CAD build for the part. Positions are in the model's coordinates, mm. A direction names the side the tool comes from. Round coordinates to 2 decimals unless told otherwise and drop trailing zeros. Loops run counter-clockwise (first coordinate to the right, second up) from the corner with the lowest first, then second, coordinate; pieces in that order, holes last. Notation, with made-up numbers: (-3, 39) - (30, 39) arc R20 cw to (30, 55) - close; hole circle Ø11 at (1, 65.5). An arc over 180 degrees is marked (long way). One line per question, with ' | ' between items.
```python
from build123d import *

# Parameters (mm, degrees)
SKETCH1_W                                      = 200
SKETCH1_H                                      = 174.75
BOSS_EXTRUDE1_DEPTH                            = 25
SKETCH2_W                                      = 40
SKETCH2_H                                      = 9.75
CUT_EXTRUDE1_DEPTH                             = 19.8
SKETCH3_W                                      = 37.5
SKETCH3_H                                      = 60
CUT_EXTRUDE2_DEPTH                             = 26
BOSS_EXTRUDE2_DEPTH                            = 25
SKETCH5_R                                      = 1.65
CUT_EXTRUDE3_DEPTH                             = 1.23
SKETCH6_R                                      = 3.325
CUT_EXTRUDE4_DEPTH                             = 26
SKETCH7_R                                      = 0.685
CUT_EXTRUDE5_DEPTH                             = 6.2
F_1_4_20_TAPPED_HOLE1_D                        = 5.1054
CBORE_FOR_4_SOCKET_HEAD_CAP_SCREW1_D           = 3.2639
CBORE_FOR_4_SOCKET_HEAD_CAP_SCREW1_CBORE_D     = 5.55752
CBORE_FOR_4_SOCKET_HEAD_CAP_SCREW1_CBORE_DEPTH = 2.8448


with BuildPart() as part:
    # Sketch1 → Boss-Extrude1 (new body)
    with BuildSketch(Plane(origin=(0, 0, 0), x_dir=(1, 0, 0), z_dir=(0, 1, 0))):
        Rectangle(SKETCH1_W, SKETCH1_H)
    extrude(amount=BOSS_EXTRUDE1_DEPTH)

    # Sketch2 → Cut-Extrude1 (cut)
    with BuildSketch(Plane(origin=(0, 25, 0), x_dir=(1, 0, 0), z_dir=(0, 1, 0))):
        with Locations((-80, -82.5)):
            Rectangle(SKETCH2_W, SKETCH2_H)
    extrude(amount=-CUT_EXTRUDE1_DEPTH, mode=Mode.SUBTRACT)

    # Sketch3 → Cut-Extrude2 (cut, through all)
    with BuildSketch(Plane(origin=(0, 25, 0), x_dir=(1, 0, 0), z_dir=(0, 1, 0))):
        with Locations((-79.98, -42.625)):
            Rectangle(SKETCH3_W, SKETCH3_H)
        Polygon((-25, -42.625), (100, -42.625), (100, -87.375), (-60, -87.375), (-60, -12.625), (-25, -12.625), align=None)
    extrude(amount=-CUT_EXTRUDE2_DEPTH, mode=Mode.SUBTRACT)

    # Sketch4 → Boss-Extrude2 (add)
    with BuildSketch(Plane(origin=(0, 25, 0), x_dir=(1, 0, 0), z_dir=(0, 1, 0))):
        Polygon((-60, -74.625), (-5.5, -74.625), (-5.5, -73.455), (-50.1, -73.455), (-50.1, -69.865), (49.9, -69.865), (49.9, -73.455), (5.2, -73.455), (5.2, -74.625), (59.7, -74.625), (59.7, -75.855), (5.2, -75.855), (5.2, -77.025), (49.9, -77.025), (49.9, -80.615), (-50.1, -80.615), (-50.1, -77.025), (-5.5, -77.025), (-5.5, -75.855), (-60, -75.855), align=None)
        Polygon((-3.1, -72.225), (-3.1, -78.255), (-47.63, -78.255), (-47.63, -79.385), (47.43, -79.385), (47.43, -78.255), (2.8, -78.255), (2.8, -72.225), (47.43, -72.225), (47.43, -71.095), (-47.63, -71.095), (-47.63, -72.225), align=None, mode=Mode.SUBTRACT)
    extrude(amount=-BOSS_EXTRUDE2_DEPTH)

    # Sketch5 → Cut-Extrude3 (cut)
    with BuildSketch(Plane.XY.offset(75.855)):
        with Locations((54.55, 12.65)):
            Circle(SKETCH5_R)
    extrude(amount=-CUT_EXTRUDE3_DEPTH, mode=Mode.SUBTRACT)

    # Sketch6 → Cut-Extrude4 (cut, through all)
    with BuildSketch(Plane(origin=(0, 25, 0), x_dir=(1, 0, 0), z_dir=(0, 1, 0))):
        with Locations((-80.175, 67.55)):
            Circle(SKETCH6_R)
        with Locations((-4.025, 67.55)):
            Circle(SKETCH6_R)
        with Locations((-4.025, 16.9)):
            Circle(SKETCH6_R)
    extrude(amount=-CUT_EXTRUDE4_DEPTH, mode=Mode.SUBTRACT)

    # Sketch7 → Cut-Extrude5 (cut, through all)
    with BuildSketch(Plane(origin=(0, 5.2, 0), x_dir=(1, 0, 0), z_dir=(0, 1, 0))):
        with Locations((-92.665, -82.29)):
            Circle(SKETCH7_R)
        with Locations((-67.795, -82.29)):
            Circle(SKETCH7_R)
    extrude(amount=-CUT_EXTRUDE5_DEPTH, mode=Mode.SUBTRACT)

    # 1/4-20 Tapped Hole1 (through all)
    with Locations(Plane(origin=(0, 25, 0), x_dir=(1, 0, 0), z_dir=(0, 1, 0))):
        with Locations((51.745235504, 41.326927492), (81.748513239, 41.326927492), (81.748513239, -18.673072418), (51.745235504, -18.673072418)):
            Hole(F_1_4_20_TAPPED_HOLE1_D / 2)

    # CBORE for #4 Socket Head Cap Screw1 (through all)
    with Locations(Plane(origin=(0, 5.2, 0), x_dir=(1, 0, 0), z_dir=(0, 1, 0))):
        with Locations((-92.665, -82.29), (-67.795, -82.29)):
            CounterBoreHole(CBORE_FOR_4_SOCKET_HEAD_CAP_SCREW1_D / 2, CBORE_FOR_4_SOCKET_HEAD_CAP_SCREW1_CBORE_D / 2, CBORE_FOR_4_SOCKET_HEAD_CAP_SCREW1_CBORE_DEPTH)


solid = part.part
```
(1) Cut at D-D, the plane x = -37.5. Write the cut outline in (y, z) (3 decimals).
Results found:
outline: (0, -87.375) - (25, -87.375) - (25, 12.625) - (0, 12.625) - close; (0, 69.865) - (25, 69.865) - (25, 71.095) - (0, 71.095) - close; (0, 72.225) - (25, 72.225) - (25, 73.455) - (0, 73.455) - close; (0, 74.625) - (25, 74.625) - (25, 75.855) - (0, 75.855) - close; (0, 77.025) - (25, 77.025) - (25, 78.255) - (0, 78.255) - close; (0, 79.385) - (25, 79.385) - (25, 80.615) - (0, 80.615) - close
(2) Probe L1, parallel to Z at x = 38.5, y = 10.25 (3 decimals); L2, parallel to Z at x = -27, y = 7 (3 decimals); L3, parallel to X at y = 11, z = -41.5. List the from-to ranges inside material, lowest first.
Results found:
L1: z = -87.375 to 42.625, 69.865 to 71.095, 72.225 to 73.455, 74.625 to 75.855, 77.025 to 78.255, 79.385 to 80.615 | L2: z = -87.375 to 12.625, 69.865 to 71.095, 72.225 to 73.455, 74.625 to 75.855, 77.025 to 78.255, 79.385 to 80.615 | L3: x = -100 to 49.2, 54.29 to 79.2, 84.3 to 100
(3) Cut at A-A, the plane z = -16.9. Write the cut outline in (x, y).
Results found:
outline: (-100, 0) - (-7.35, 0) - (-7.35, 25) - (-100, 25) - close; (-0.7, 0) - (100, 0) - (100, 25) - (-0.7, 25) - close
(4) Tool access for faces 1 (the face through (-80, 15, 77.625)), 2 (the face through (37, 13, 42.625)), 3 (the face through (-43, 13, 12.625)): list every direction of +Z, -Z, +X, -X, +Y, -Y with a clear straight run to the whole face (end or side of a thin tool).
Results found:
face 1: +Z, -X, +Y | face 2: +X, +Y, -Y | face 3: +Y, -Y
(5) Drop flat-ended pins along their axis: P1, Ø7.5, axis at x = -17.5, y = 13.5, coming from the +Z side (3 decimals); P2, Ø4, axis at y = 12, z = 78.5, coming from the +X side; P3, Ø4.5, axis at x = -92.665, z = 82.29, coming from the -Y side; P4, Ø1.7, axis at x = -91.5, z = 82, coming from the +Y side. Give the stop position or say it passes through.
Results found:
P1: stops at z = 80.615 | P2: stops at x = 49.9 | P3: stops at y = 0 | P4: stops at y = 2.36
(6) Two-plate mould, pull along X, no slides. Class faces 4 (the face through (-100, 12, 1)), 5 (the face through (54.295, 12.325, 18.561)), 6 (the face through (-80, 3, 87.375)), 7 (the face through (54.295, 12.325, -41.439)): released by +X, released by -X, zero draft, split by the parting line, or undercut.
Results found:
face 4: released by -X | face 5: undercut | face 6: zero draft | face 7: undercut
(7) Cut at C-C, the plane z = 26. Write the cut outline in (x, y).
Results found:
outline: (-100, 0) - (-98.73, 0) - (-98.73, 25) - (-100, 25) - close; (-61.23, 0) - (-60, 0) - (-60, 25) - (-61.23, 25) - close; (-25, 0) - (100, 0) - (100, 25) - (-25, 25) - close
(8) Cut at B-B, the plane x = 20. Write the cut outline in (y, z) (3 decimals), then the cut area to 3 significant figures.
Results found:
outline: (0, -87.375) - (25, -87.375) - (25, 42.625) - (0, 42.625) - close; (0, 69.865) - (25, 69.865) - (25, 71.095) - (0, 71.095) - close; (0, 72.225) - (25, 72.225) - (25, 73.455) - (0, 73.455) - close; (0, 74.625) - (25, 74.625) - (25, 75.855) - (0, 75.855) - close; (0, 77.025) - (25, 77.025) - (25, 78.255) - (0, 78.255) - close; (0, 79.385) - (25, 79.385) - (25, 80.615) - (0, 80.615) - close | area: 3,400 mm²
